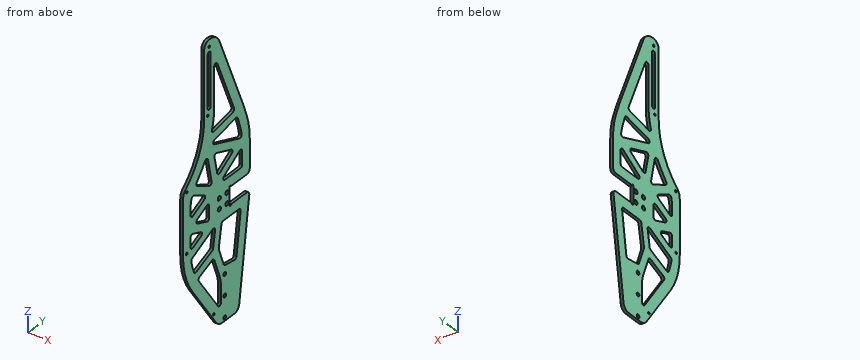
```python
from build123d import *

# Parameters (mm, degrees)
SKETCH2_R               = 3.125
SKETCH2_R_2             = 1.625
BOSS_EXTRUDE1_DEPTH     = 4
SKETCH4_R               = 2.625
CUT_EXTRUDE1_DEPTH      = 4
CUT_EXTRUDE2_DEPTH      = 4
CUT_EXTRUDE3_DEPTH      = 251.422576691
CUT_EXTRUDE3_DEPTH_BACK = 10
FILLET1_START           = -1
FILLET1_DEPTH           = 6
FILLET2_R               = 15
FILLET3_R               = 3.175


with BuildPart() as part:
    # Sketch2 → Boss-Extrude1 (new body)
    with BuildSketch(Plane(origin=(0, 0, 0), x_dir=(0, 0, -1), z_dir=(1, 0, 0))):
        with BuildLine():
            Line((-12.5, 12.5), (12.5, 12.5))
            ThreePointArc((12.5, 12.5), (14, 14), (12.5, 15.5))
            Line((12.5, 15.5), (12.5, 46.748157964))
            ThreePointArc((12.5, 46.748157964), (14.219704855, 50.521705865), (18.195865505, 51.699498308))
            Line((18.195865505, 51.699498308), (158.89173101, 31.92598393))
            ThreePointArc((158.89173101, 31.92598393), (165.047095802, 28.583893533), (167.5, 22.023303243))
            Line((167.5, 22.023303243), (167.5, -9.283829379))
            Line((167.5, -9.283829379), (93.327764747, -61.219787629))
            ThreePointArc((93.327764747, -61.219787629), (66.040701063, -74.676278275), (35.970121112, -79.3045832))
            Line((35.970121112, -79.3045832), (-50.348010792, -79.3045832))
            ThreePointArc((-50.348010792, -79.3045832), (-85.935359672, -48.630118411), (-131.603387734, -37.593207459))
            Line((-131.603387734, -37.593207459), (-227.5, -37.593207459))
            ThreePointArc((-227.5, -37.593207459), (-234.571067812, -34.664275271), (-237.5, -27.593207459))
            Line((-237.5, -27.593207459), (-237.5, -25.880734277))
            ThreePointArc((-237.5, -25.880734277), (-234.158594281, -14.813158364), (-225.250876341, -7.443708597))
            Line((-225.250876341, -7.443708597), (-112.5, 39.956458601))
            Line((-112.5, 39.956458601), (-94.069316262, 46.664678879))
            ThreePointArc((-94.069316262, 46.664678879), (-77.232119696, 51.176192101), (-59.867301929, 52.6954168))
            Line((-59.867301929, 52.6954168), (-17.5, 52.6954168))
            ThreePointArc((-17.5, 52.6954168), (-13.964466094, 51.230950706), (-12.5, 47.6954168))
            Line((-12.5, 47.6954168), (-12.5, 15.5))
            ThreePointArc((-12.5, 15.5), (-14, 14), (-12.5, 12.5))
        make_face()
        with Locations((-7.5, 7.5)):
            Circle(SKETCH2_R, mode=Mode.SUBTRACT)
        with Locations((7.5, 7.5)):
            Circle(SKETCH2_R, mode=Mode.SUBTRACT)
        with Locations((7.5, -7.5)):
            Circle(SKETCH2_R, mode=Mode.SUBTRACT)
        with Locations((-7.5, -7.5)):
            Circle(SKETCH2_R, mode=Mode.SUBTRACT)
        with Locations((-227.5, -27.593207459)):
            Circle(SKETCH2_R_2, mode=Mode.SUBTRACT)
        with Locations((-133.504211585, -30.116786314)):
            Circle(SKETCH2_R_2, mode=Mode.SUBTRACT)
        with Locations((-49.002692564, -71.8045832)):
            Circle(SKETCH2_R_2, mode=Mode.SUBTRACT)
        with Locations((35.970121112, -72.097727652)):
            Circle(SKETCH2_R_2, mode=Mode.SUBTRACT)
        with Locations((147.103987767, -18.332333959)):
            Circle(SKETCH2_R_2, mode=Mode.SUBTRACT)
    extrude(amount=BOSS_EXTRUDE1_DEPTH)

    # Sketch4 → Cut-Extrude1 (cut)
    with BuildSketch(Plane(origin=(4, 0, 0), x_dir=(0, 0, -1), z_dir=(1, 0, 0))):
        with Locations((102.5, 3.216170621)):
            Circle(SKETCH4_R)
        with Locations((162.5, 3.216170621)):
            Circle(SKETCH4_R)
        with Locations((132.5, 3.216170621)):
            Circle(SKETCH4_R)
    extrude(amount=-CUT_EXTRUDE1_DEPTH, mode=Mode.SUBTRACT)

    # Sketch7 → Cut-Extrude2 (cut)
    with BuildSketch(Plane.ZY):
        with BuildLine():
            Line((143.504211585, -24.593207459), (217.5, -24.593207459))
            ThreePointArc((217.5, -24.593207459), (220.5, -27.593207459), (217.5, -30.593207459))
            Line((217.5, -30.593207459), (143.504211585, -30.593207459))
            ThreePointArc((143.504211585, -30.593207459), (140.504211585, -27.593207459), (143.504211585, -24.593207459))
        make_face()
    extrude(amount=-CUT_EXTRUDE2_DEPTH, mode=Mode.SUBTRACT)

    # Sketch8 → Cut-Extrude3 (cut, two sides: drawn at the far end of the back side and taken through both)
    with BuildSketch(Plane(origin=(4, 0, 0), x_dir=(0, 0, -1), z_dir=(1, 0, 0)).offset(-CUT_EXTRUDE3_DEPTH_BACK)):
        with BuildLine():
            Line((-113.57117516, 23.234534385), (-210.688209636, -17.593207459))
            Line((-210.688209636, -17.593207459), (-139.249392001, -17.593207459))
            ThreePointArc((-139.249392001, -17.593207459), (-128.305621954, -18.193841781), (-117.493315985, -19.988529516))
            ThreePointArc((-117.493315985, -19.988529516), (-110.906374998, -21.611191224), (-104.398029564, -23.524895038))
            Line((-104.398029564, -23.524895038), (-113.57117516, 23.234534385))
        make_face()
        with BuildLine():
            ThreePointArc((-38.896111202, -61.219787629), (-31.347289926, -63.525803076), (-23.492615431, -64.3045832))
            Line((-23.492615431, -64.3045832), (-7.844578132, -64.3045832))
            Line((-7.844578132, -64.3045832), (-23.897236503, -31.471478495))
            Line((-23.897236503, -31.471478495), (-38.896111202, -61.219787629))
        make_face()
        with BuildLine():
            Line((82.520271866, -50.475656782), (148.489038099, -4.283829379))
            Line((148.489038099, -4.283829379), (116.676340901, -4.283829379))
            ThreePointArc((116.676340901, -4.283829379), (107.646731671, -5.091144924), (98.911316911, -7.515630477))
            Line((98.911316911, -7.515630477), (69.575731894, -18.680359782))
            Line((69.575731894, -18.680359782), (82.520271866, -50.475656782))
        make_face()
        Polygon((90.339984209, 2.061933427), (93.696000857, 25.941232677), (27.5, 35.244473892), (27.5, -2.831339099), (62.03978176, -8.708743191), align=None)
        Polygon((-27.5, -7.735456644), (-27.5, 37.6954168), (-55.598162704, 37.6954168), align=None)
        with BuildLine():
            Line((-88.939014112, 32.569289567), (-102.31343439, 28.184098276))
            Line((-102.31343439, 28.184098276), (-91.212566173, -28.401754251))
            Line((-91.212566173, -28.401754251), (-67.955274479, 37.309745965))
            ThreePointArc((-67.955274479, 37.309745965), (-78.597719011, 35.60604022), (-88.939014112, 32.569289567))
        make_face()
        Polygon((13.776543649, -27.5), (-12.481500104, -27.5), (2.390501596, -57.918263299), align=None)
        Polygon((-74.89478187, -18.263165558), (-39.778603589, -10.696041624), (-60.41005824, 22.662189485), align=None)
        with BuildLine():
            Line((-49.181599521, -54.965243604), (-37.325171166, -31.449566394))
            Line((-37.325171166, -31.449566394), (-31.703807854, -21.231467759))
            Line((-31.703807854, -21.231467759), (-79.948761535, -31.627688578))
            ThreePointArc((-79.948761535, -31.627688578), (-66.849258357, -40.525120988), (-54.439866562, -50.362208069))
            Line((-54.439866562, -50.362208069), (-50.683815172, -53.641226781))
            ThreePointArc((-50.683815172, -53.641226781), (-49.940993749, -54.312636858), (-49.181599521, -54.965243604))
        make_face()
        Polygon((23.060748964, -36.927651205), (12.81312582, -64.3045832), (35.970121112, -64.3045832), align=None)
        with BuildLine():
            Line((25.857837049, -14.724396782), (48.779257286, -63.333899694))
            ThreePointArc((48.779257286, -63.333899694), (60.611766088, -60.654379345), (71.942273955, -56.317596515))
            Line((71.942273955, -56.317596515), (57.178612381, -20.054044039))
            Line((57.178612381, -20.054044039), (25.857837049, -14.724396782))
        make_face()
    extrude(amount=CUT_EXTRUDE3_DEPTH + CUT_EXTRUDE3_DEPTH_BACK, mode=Mode.SUBTRACT)

    # Fillet1: read off the stored shape, not the designer's step
    # Fillet1 outline → Fillet1 (cut)
    with BuildSketch(Plane.YZ.offset(FILLET1_START)):
        with BuildLine():
            Line((-79.3045832, 50.348010792), (-79.3045832, 40.658946938))
            add(Edge.make_bspline(
                [(-79.3045832, 40.658946938), (-79.3045832, 42.329655762), (-79.3045832, 44.000364586), (-78.966879258, 47.665805706), (-77.514803195, 50.954845241), (-74.76186007, 53.781947885), (-73.525620436, 54.806645775), (-72.352687243, 55.816353737)],
                knots=[0, 0, 0, 0, 0, 0, 0.5, 0.5, 1, 1, 1, 1, 1, 1], degree=5))
            ThreePointArc((-72.352687243, 55.816353737), (-75.76814719, 53.005283923), (-79.3045832, 50.348010792))
        make_face()
    extrude(amount=FILLET1_DEPTH, mode=Mode.SUBTRACT)

    # Fillet2
    fillet2_edges = [part.edges().sort_by_distance(p)[0] for p in [
        (2, -9.283829379, -167.5),
    ]]
    fillet(fillet2_edges, radius=FILLET2_R)

    # Fillet3
    fillet3_edges = [part.edges().sort_by_distance(p)[0] for p in [
        (2, -17.593207459, 210.688209636),
        (2, 37.309745965, 67.955274479),
        (2, -7.735456644, 27.5),
        (2, 37.6954168, 55.598162704),
        (2, 37.6954168, 27.5),
        (2, -18.263165558, 74.89478187),
        (2, -31.627688578, 79.948761535),
        (2, -21.231467759, 31.703807854),
        (2, -54.965243604, 49.181599521),
        (2, -61.219787629, 38.896111202),
        (2, -64.3045832, 7.844578132),
        (2, -31.471478495, 23.897236503),
        (2, -57.918263299, -2.390501596),
        (2, -27.5, -13.776543649),
        (2, -27.5, 12.481500104),
        (2, -64.3045832, -12.81312582),
        (2, -36.927651205, -23.060748964),
        (2, -64.3045832, -35.970121112),
        (2, -14.724396782, -25.857837049),
        (2, -20.054044039, -57.178612381),
        (2, -63.333899694, -48.779257286),
        (2, -56.317596515, -71.942273955),
        (2, -50.475656782, -82.520271866),
        (2, -4.283829379, -148.489038099),
        (2, -18.680359782, -69.575731894),
        (2, -2.831339099, -27.5),
        (2, -8.708743191, -62.03978176),
        (2, 2.061933427, -90.339984209),
        (2, 25.941232677, -93.696000857),
        (2, 35.244473892, -27.5),
        (2, -10.696041624, 39.778603589),
        (2, -28.401754251, 91.212566173),
        (2, 28.184098276, 102.31343439),
        (2, 22.662189485, 60.41005824),
        (2, -23.524895038, 104.398029564),
        (2, 23.234534385, 113.57117516),
    ]]
    fillet(fillet3_edges, radius=FILLET3_R)


solid = part.part
```
Verification items for the finished model (mm, model axes). Round coordinates to 2 decimals unless told otherwise and drop trailing zeros. Order: outer loops, then holes, each group sorted by start corner. A loop starts at its lowest first (then second) coordinate and runs counter-clockwise, first axis right, second up. Notation, with made-up numbers: (49.25, 23.25) - (107.25, 23.25) arc R14 ccw to (107.25, 27.25) - close; hole circle Ø10 at (10, -25.5). An arc over 180 degrees is marked (long way). Use CSV: the item, a comma, the result in double quotes. Start each with the question number.
1) Thickness scan on L1, parallel to Y at x = 2.95, z = 174; L2, parallel to Z at x = 1.3, y = 23; L3, parallel to Y at x = 0.8, z = 55. Record the ranges inside material, lowest first.
2) Section check B-B, the plane x = 1.55. State how many separate pieces and enclosed holes the cut face has, plus the area to 3 significant figures.
3) Section check A-A, the plane z = 151.5. Record the cut outline in (x, y).
4) Go/stop test with flat-tipped pins: P1, Ø1.5, axis at x = 1.5, z = -58.5, coming from the +Y side; P2, Ø1, axis at x = 1, z = 77, coming from the -Y side; P3, Ø1.5, axis at x = 0.5, z = -105.5, coming from the -Y side. Record where each tip stops, or that it passes through.
Answers:
1,L1,"y = -37.59 to -30.59, -24.59 to -17.59, -2.17 to 14.1"
1,L2,"z = -167.45 to -93.28, -27.5 to -12.5, 12.5 to 27.5, 46.51 to 73.02, 101.3 to 152.83"
1,L3,"y = -73.3 to -49.89, -26.25 to -13.98, 13.91 to 52.7"
2,separate pieces,"1"
2,enclosed holes,"24"
2,area,"23,100 mm²"
3,outline,"(0, -37.59) - (4, -37.59) - (4, -30.59) - (0, -30.59) - close; (0, -24.59) - (4, -24.59) - (4, -17.59) - (0, -17.59) - close; (0, 7.29) - (4, 7.29) - (4, 23.56) - (0, 23.56) - close"
4,P1,"stops at y = 46.14"
4,P2,"stops at y = -54.14"
4,P3,"stops at y = -53.22"
